The listing builds one solid part. Answer for the finished solid, in the listing's coordinates (mm). A direction names the side the tool comes from. Coordinates: 2 decimals unless noted, no trailing zeros. Order: outer loops, then holes, each group sorted by start corner. A loop starts at its lowest first (then second) coordinate and runs counter-clockwise, first axis right, second up. Notation, with made-up numbers: (32.5, 28.25) -> (89.5, 28.25) arc R32 cw to (89.5, 65.25) -> close; hole circle Ø4 at (73.25, 62). An arc over 180 degrees is marked (long way). Write item = value, one per line.
from build123d import *

# Parameters (mm, degrees)
EXTRUDE_1_DEPTH          = 275
CUT_EXTRUDE_1_DEPTH      = 276.816968296
CUT_EXTRUDE_1_DEPTH_BACK = 276.816968296
SKETCH_2_R               = 2


with BuildPart() as part:
    # 草图1 → 凸台-拉伸1 (new, symmetric)
    with BuildSketch(Plane(origin=(0, 0, 0), x_dir=(1, 0, 0), z_dir=(0, 1, 0))):
        with BuildLine():
            Line((-11, -15), (11, -15))
            ThreePointArc((11, -15), (13.828427125, -13.828427125), (15, -11))
            Line((15, -11), (15, 11))
            ThreePointArc((15, 11), (13.828427125, 13.828427125), (11, 15))
            Line((11, 15), (-11, 15))
            ThreePointArc((-11, 15), (-13.828427125, 13.828427125), (-15, 11))
            Line((-15, 11), (-15, -11))
            ThreePointArc((-15, -11), (-13.828427125, -13.828427125), (-11, -15))
        make_face()
        with BuildLine():
            Line((-11, -13), (11, -13))
            ThreePointArc((11, -13), (12.414213562, -12.414213562), (13, -11))
            Line((13, -11), (13, 11))
            ThreePointArc((13, 11), (12.414213562, 12.414213562), (11, 13))
            Line((11, 13), (-11, 13))
            ThreePointArc((-11, 13), (-12.414213562, 12.414213562), (-13, 11))
            Line((-13, 11), (-13, -11))
            ThreePointArc((-13, -11), (-12.414213562, -12.414213562), (-11, -13))
        make_face(mode=Mode.SUBTRACT)
    extrude(amount=EXTRUDE_1_DEPTH, both=True)

    # 草图2 → 切除-拉伸1 (cut, two sides: drawn at the far end of the back side and taken through both)
    with BuildSketch(Plane.XY.offset(-CUT_EXTRUDE_1_DEPTH_BACK)):
        with Locations((0, 265)):
            Circle(SKETCH_2_R)
        with Locations((0, 100)):
            Circle(SKETCH_2_R)
        with Locations((0, -100)):
            Circle(SKETCH_2_R)
        with Locations((0, -265)):
            Circle(SKETCH_2_R)
    extrude(amount=CUT_EXTRUDE_1_DEPTH + CUT_EXTRUDE_1_DEPTH_BACK, mode=Mode.SUBTRACT)


solid = part.part
Q1. A tool of negligible diameter and unlimited length cuts with its end or side. For faces 4 (the face through (13, 4, 0)), 5 (the face through (15, 4, 0)), from which of +Z, -Z, +X, -X, +Y, -Y can it reach the whole face along a straight path? Write none if from no direction.
The answers:
face_4 = +Y, -Y
face_5 = +Z, -Z, +X, +Y, -Y
Q2. This flat-tipped pin is pushed along its axis until it touches: pin 1 Ø3.5 at (x, y) = (0, 100) entering from +Z. Where does it stop, or does it pass through?
The answers:
pin_1 = through
Q3. The mould has two halves that part along Z. Classify faces 1 (the face through (0, 4, 15)), 2 (the face through (-15, 4, 0)), 3 (the face through (0, 4, 13)): released by +Z, released by -Z, zero draft, split by the parting line, or undercut.
The answers:
face_1 = released by +Z
face_2 = zero draft
face_3 = undercut
Q4. Find the intervals of material crossed by line 1 along Y through (x, z) = (0, 13.8); line 2 along Z through (x, y) = (6, -147); line 3 along X through (y, z) = (129.5, -11.5), in increasing order.
The answers:
line_1 = -275 to -267, -263 to -102, -98 to 98, 102 to 263, 267 to 275
line_2 = -15 to -13, 13 to 15
line_3 = -14.97 to -12.94, 12.94 to 14.97
Q5. Section A-A, the plane z = 5 is taken. Give the vertices of the cut face in (x, y).
The answers:
outline = (-15, -275) -> (-13, -275) -> (-13, 275) -> (-15, 275) -> close; (13, -275) -> (15, -275) -> (15, 275) -> (13, 275) -> close
Q6. Section B-B, the plane y = 219.5 is taken. Give the vertices of the cut face in (x, z), plus the area to 3 significant figures.
The answers:
outline = (-15, -11) arc R4 ccw to (-11, -15) -> (11, -15) arc R4 ccw to (15, -11) -> (15, 11) arc R4 ccw to (11, 15) -> (-11, 15) arc R4 ccw to (-15, 11) -> close; hole (-13, -11) arc R2 ccw to (-11, -13) -> (11, -13) arc R2 ccw to (13, -11) -> (13, 11) arc R2 ccw to (11, 13) -> (-11, 13) arc R2 ccw to (-13, 11) -> close
area = 214 mm2
